from build123d import *

# Parameters (mm, degrees)
SKETCH1_W               = 38
SKETCH1_H               = 11
SKETCH1_W_2             = 35
SKETCH1_H_2             = 8
BOSS_EXTRUDE1_DEPTH     = 592
CUT_EXTRUDE1_DEPTH      = 1
CUT_EXTRUDE1_DEPTH_BACK = 39
CUT_EXTRUDE3_DEPTH      = 1
CUT_EXTRUDE3_DEPTH_BACK = 39


with BuildPart() as part:
    # Sketch1 → Boss-Extrude1 (new body)
    with BuildSketch(Plane(origin=(0, 0, 0), x_dir=(0, 0, -1), z_dir=(1, 0, 0))):
        Rectangle(SKETCH1_W, SKETCH1_H)
        Rectangle(SKETCH1_W_2, SKETCH1_H_2, mode=Mode.SUBTRACT)
    extrude(amount=BOSS_EXTRUDE1_DEPTH)

    # Sketch2 → Cut-Extrude1 (cut, two sides)
    with BuildSketch(Plane(origin=(0, 0, -19), x_dir=(-1, 0, 0), z_dir=(0, 0, -1))) as cut_extrude1_sk:
        Polygon((844.430011157, 849.930011157), (0, 5.5), (-11, -5.5), (-855.430011157, -849.930011157), (833.430011157, -2538.790033471), (2533.290033471, -838.930011157), align=None)
    extrude(amount=CUT_EXTRUDE1_DEPTH, mode=Mode.SUBTRACT)
    extrude(cut_extrude1_sk.sketch, amount=-CUT_EXTRUDE1_DEPTH_BACK, mode=Mode.SUBTRACT)

    # Sketch3 → Cut-Extrude3 (cut, two sides)
    with BuildSketch(Plane(origin=(0, 0, -19), x_dir=(-1, 0, 0), z_dir=(0, 0, -1))) as cut_extrude3_sk:
        Polygon((-1436.430011157, 849.930011157), (-592, 5.5), (-581, -5.5), (263.430011157, -849.930011157), (-1425.430011157, -2538.790033471), (-3125.290033471, -838.930011157), align=None)
    extrude(amount=CUT_EXTRUDE3_DEPTH, mode=Mode.SUBTRACT)
    extrude(cut_extrude3_sk.sketch, amount=-CUT_EXTRUDE3_DEPTH_BACK, mode=Mode.SUBTRACT)


solid = part.part
Can you work these out from the model? Positions are in its coordinate system, mm. A direction names the side the tool comes from. Round coordinates to 2 decimals unless told otherwise and drop trailing zeros. Loops run counter-clockwise (first coordinate to the right, second up) from the corner with the lowest first, then second, coordinate; pieces in that order, holes last. Notation, with made-up numbers: (89, -1.75) - (139, -1.75) arc R18 ccw to (139, 28.25) - close; hole circle Ø7 at (85, 24). An arc over 180 degrees is marked (long way). Use CSV: the item, a comma, the result in double quotes. Start each with the question number.
1) If we section it at C-C on x = 429.5: Write out the boundary of the cut face in (y, z), plus the area to 3 significant figures.
2) Please list where these lines run through material, in increasing order: probe 1 along Y at (x, z) = (27.5, 9.5); probe 2 along Z at (x, y) = (427, -3.75); probe 3 along X at (y, z) = (-4.5, 7). Write a range as [from, to].
3) If we section it at A-A on y = -0.5: Write out the boundary of the cut face in (x, z).
4) For faces 1 (the flat face through (292, -5.5, 0)), 2 (the flat face through (292, -4, 0)), which set-ups out of +Z, -Z, +X, -X, +Y, -Y let a thin tool reach every point of the face, with its end or its side?
5) If we section it at B-B on z = -9.5: Write out the boundary of the cut face in (x, y).
6) We'd pull the mould along Z, two halves only. Please class faces 3 (the flat face through (292, 0, 19)), 4 (the flat face through (292, 0, -19)), 5 (the flat face through (292, 4, 0)), 6 (the flat face through (582, -4.5, 2.7)): released by +Z, released by -Z, zero draft, split by the parting line, or undercut.
Geometry results:
1,outline,"(-5.5, -19) - (5.5, -19) - (5.5, 19) - (-5.5, 19) - close; hole (-4, -17.5) - (4, -17.5) - (4, 17.5) - (-4, 17.5) - close"
1,area,"138 mm2"
2,probe 1,"y = [-5.5, -4], [4, 5.5]"
2,probe 2,"z = [-19, -17.5], [17.5, 19]"
2,probe 3,"x = [10, 582]"
3,outline,"(6, -19) - (586, -19) - (586, -17.5) - (6, -17.5) - close; (6, 17.5) - (586, 17.5) - (586, 19) - (6, 19) - close"
4,face 1,"+Z, -Z, +X, -X, -Y"
4,face 2,"+X, -X"
5,outline,"(0, 5.5) - (1.5, 4) - (590.5, 4) - (592, 5.5) - close; (9.5, -4) - (11, -5.5) - (581, -5.5) - (582.5, -4) - close"
6,face 3,"released by +Z"
6,face 4,"released by -Z"
6,face 5,"undercut"
6,face 6,"zero draft"
